Can you work these out from the drawing? Everything is in mm from the part's minimum corner. A direction names the side the tool comes from. Give positions to 0.01 mm unless a question says otherwise; leave off trailing zeros. Loops run counter-clockwise (first coordinate to the right, second up) from the corner with the lowest first, then second, coordinate; pieces in that order, holes last.
Q1. If we section it at A-A (x = 29): Please give me the cut outline in (y, z) (1 decimal).
Q2. If we section it at D-D (x = 74.5): Please give me the cut outline in (y, z).
Q3. We'd pull the mould along X, two halves only. Please class the marked faces 1, 2 and 3: +X half, -X half, draft (parallel to the pull), parting line (faces both ways), or undercut.
Q4. I need wall thicknesses on line 1 (X direction, y = 39.5, z = 29.5) (1 decimal); line 2 (X direction, y = 28, z = 15.5) (1 decimal); line 3 (Y direction, x = 59, z = 41) (1 decimal). Which ranges of each line are inside material? Lowest first, please.
Q5. If we section it at B-B (y = 38.5): Please give me the cut outline in (x, z) (1 decimal), plus the area to 3 significant figures.
Q6. For the marked faces 4 and 5, which set-ups out of +Z, -Z, +X, -X, +Y, -Y let a thin tool reach every point of the face, with its end or its side?
Q7. If we section it at C-C (z = 35.5): Please give me the cut outline in (x, y) (1 decimal).
Q8. Will these pins go through, and if not, where does the flat tip stop? P1, Ø2, axis at x = 21, z = 53.5, coming from the +Y side; P2, Ø10, axis at x = 13, z = 46, coming from the -Y side; P3, Ø4, axis at x = 42.5, z = 16.5, coming from the -Y side.
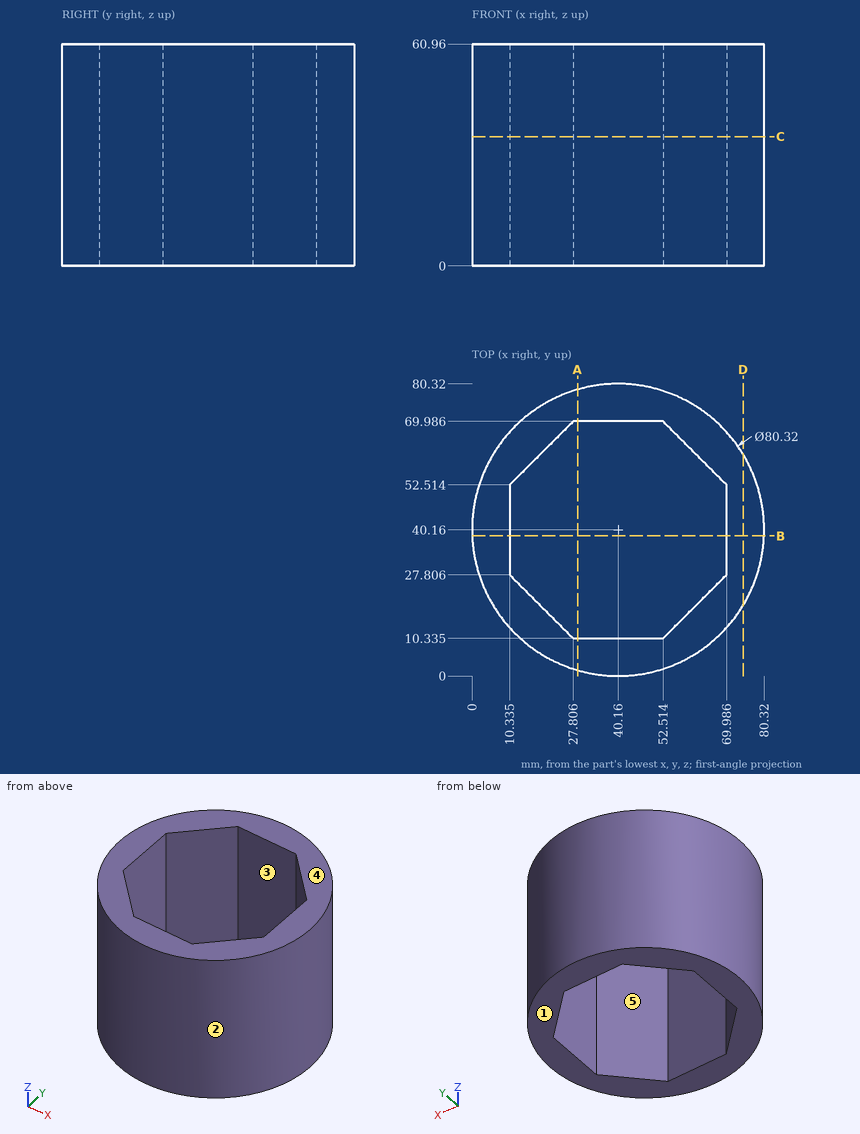
Check sheet entries:
1. outline: (1.6, 0) - (10.3, 0) - (10.3, 61) - (1.6, 61) - close; (70, 0) - (78.7, 0) - (78.7, 61) - (70, 61) - close
2. outline: (19.34, 0) - (60.98, 0) - (60.98, 60.96) - (19.34, 60.96) - close
3. face 1: draft
3. face 2: parting line
3. face 3: undercut
4. line 1: x = 0 to 10.3, 70 to 80.3
4. line 2: x = 1.9 to 10.3, 70 to 78.4
4. line 3: y = 4.7 to 16.8, 63.5 to 75.6
5. outline: (0, 0) - (10.3, 0) - (10.3, 61) - (0, 61) - close; (70, 0) - (80.3, 0) - (80.3, 61) - (70, 61) - close
5. area: 1,260 mm2
6. face 4: +Z, +X, -X, +Y, -Y
6. face 5: +Z, -Z
7. outline: circle Ø80.3 at (40.2, 40.2); hole (10.3, 27.8) - (27.8, 10.3) - (52.5, 10.3) - (70, 27.8) - (70, 52.5) - (52.5, 70) - (27.8, 70) - (10.3, 52.5) - close
8. P1: stops at y = 75.98
8. P2: stops at y = 6.67
8. P3: stops at y = 0
